Input: part model. Units: mm. Frame: model coordinates. A direction names the side the tool comes from. Coordinates: 2 decimals unless noted, no trailing zeros. Write each loop counter-clockwise with the first axis right and the second up, starting at its lowest first coordinate (ties: lowest second). Pieces come first, ordered by that corner, then holes. Notation, with made-up numbers: M -17.5,4 L 16.5,4 A33 ccw 16.5,36 Z; hole C 9,-5 d3. An arc over 180 degrees is marked long. Use CSV: the item, a comma, the result in double quotes.
```python
from build123d import *

# Parameters (mm, degrees)
F0_W      = 152.0995497704
F0_H      = 153.0030965805
F1_DEPTH  = 25.4
F2_W      = 137.3413652182
F2_H      = 135.8354389668
F3_DEPTH  = 25.4
F4_W      = 120.4748898745
F4_H      = 118.9689487219
F5_DEPTH  = 25.4
F6_W      = 102.4036556482
F6_H      = 100.8977144957
F7_DEPTH  = 25.4
F8_W      = 81.9229260087
F8_H      = 84.0312317014
F9_DEPTH  = 25.4
F10_W     = 66.863566637
F10_H     = 68.3694928885
F11_DEPTH = 25.4
F12_W     = 51.2018278241
F12_H     = 53.9125055075
F13_DEPTH = 25.4
F14_W     = 34.3353450298
F14_H     = 36.4436469972
F15_DEPTH = 25.4
F15_TAPER = 5
F16_W     = 19.8783595115
F16_H     = 20.1795380563
F17_DEPTH = 25.4
F17_TAPER = 5
F18_W     = 7.8308703378
F18_H     = 6.9273011759
F19_DEPTH = 25.4
F19_TAPER = 5


with BuildPart() as f1:
    # F0 (on Front) → F1 (new body)
    with BuildSketch(Plane.XZ):
        with Locations((-0.150591135, -0.150591135)):
            Rectangle(F0_W, F0_H)
    extrude(amount=F1_DEPTH)

    # F2 (on face) → F3 (join)
    with BuildSketch(Plane.XZ.offset(25.4)):
        Rectangle(F2_W, F2_H)
    extrude(amount=F3_DEPTH)

    # F4 (on face) → F5 (join)
    with BuildSketch(Plane.XZ.offset(50.8)):
        Rectangle(F4_W, F4_H)
    extrude(amount=F5_DEPTH)

    # F6 (on face) → F7 (join)
    with BuildSketch(Plane.XZ.offset(76.2)):
        Rectangle(F6_W, F6_H)
    extrude(amount=F7_DEPTH)

    # F8 (on face) → F9 (join)
    with BuildSketch(Plane.XZ.offset(101.6)):
        Rectangle(F8_W, F8_H)
    extrude(amount=F9_DEPTH)

    # F10 (on face) → F11 (join)
    with BuildSketch(Plane.XZ.offset(127)):
        Rectangle(F10_W, F10_H)
    extrude(amount=F11_DEPTH)

    # F12 (on face) → F13 (join)
    with BuildSketch(Plane.XZ.offset(152.4)):
        Rectangle(F12_W, F12_H)
    extrude(amount=F13_DEPTH)

    # F14 (on face) → F15 (join)
    with BuildSketch(Plane.XZ.offset(177.8)):
        Rectangle(F14_W, F14_H)
    extrude(amount=F15_DEPTH, taper=F15_TAPER)

    # F16 (on face) → F17 (join)
    with BuildSketch(Plane.XZ.offset(203.2)):
        Rectangle(F16_W, F16_H)
    extrude(amount=F17_DEPTH, taper=F17_TAPER)

    # F18 (on face) → F19 (join)
    with BuildSketch(Plane.XZ.offset(228.6)):
        Rectangle(F18_W, F18_H)
    extrude(amount=F19_DEPTH, taper=F19_TAPER)


solid = f1.part
```
1. Section C-C (y = -123). Return loops of the section in (x, z).
Resolved:
outline,"M -40.96,-42.02 L 40.96,-42.02 L 40.96,42.02 L -40.96,42.02 Z"
2. Section A-A (x = -57). Return loops of the section in (y, z).
Resolved:
outline,"M -76.2,-59.48 L -50.8,-59.48 L -50.8,-67.92 L -25.4,-67.92 L -25.4,-76.65 L 0,-76.65 L 0,76.35 L -25.4,76.35 L -25.4,67.92 L -50.8,67.92 L -50.8,59.48 L -76.2,59.48 Z"
3. Section B-B (z = -23.5). Return loops of the section in (x, y), then the cut area to 3 significant figures.
Resolved:
outline,"M -76.2,-25.4 L -68.67,-25.4 L -68.67,-50.8 L -60.24,-50.8 L -60.24,-76.2 L -51.2,-76.2 L -51.2,-101.6 L -40.96,-101.6 L -40.96,-127 L -33.43,-127 L -33.43,-152.4 L -25.6,-152.4 L -25.6,-177.8 L 25.6,-177.8 L 25.6,-152.4 L 33.43,-152.4 L 33.43,-127 L 40.96,-127 L 40.96,-101.6 L 51.2,-101.6 L 51.2,-76.2 L 60.24,-76.2 L 60.24,-50.8 L 68.67,-50.8 L 68.67,-25.4 L 75.9,-25.4 L 75.9,0 L -76.2,0 Z"
area,"18,100 mm^2"
4. Section D-D (x = 22). Return loops of the section in (y, z).
Resolved:
outline,"M -177.8,-26.96 L -152.4,-26.96 L -152.4,-34.18 L -127,-34.18 L -127,-42.02 L -101.6,-42.02 L -101.6,-50.45 L -76.2,-50.45 L -76.2,-59.48 L -50.8,-59.48 L -50.8,-67.92 L -25.4,-67.92 L -25.4,-76.65 L 0,-76.65 L 0,76.35 L -25.4,76.35 L -25.4,67.92 L -50.8,67.92 L -50.8,59.48 L -76.2,59.48 L -76.2,50.45 L -101.6,50.45 L -101.6,42.02 L -127,42.02 L -127,34.18 L -152.4,34.18 L -152.4,26.96 L -177.8,26.96 Z"
5. Material intervals for line 1 (Y direction, x = -1, z = -50.5); line 2 (Z direction, x = 47.5, y = -47.5); line 3 (X direction, y = -111, z = 32.5), sorted ascending. Write a range as [from, to].
Resolved:
line 1,"y = [-76.2, 0]"
line 2,"z = [-67.92, 67.92]"
line 3,"x = [-40.96, 40.96]"
6. Contact query for flat-ended pins moving along their axis: pin 1 Ø12.5 at (x, y) = (-15.5, -86) entering from -Z; pin 2 Ø7.5 at (y, z) = (-134, -6) entering from +X; pin 3 Ø12.5 at (y, z) = (-143.5, 1.5) entering from -X. Output: stop coordinate, or through.
Resolved:
pin 1,"stops at z = -50.45"
pin 2,"stops at x = 33.43"
pin 3,"stops at x = -33.43"
7. Access query for faces 1 (the flat face through (-40.961, -114, -1)), 2 (the flat face through (51.202, -89, -1)), 3 (the flat face through (0, -140, -34.185)). Directions: +Z, -Z, +X, -X, +Y, -Y. A direction counts if a zero-diameter tool reaches every point of the face in a straight line with its end or side. Return the directions, or none.
Resolved:
face 1,"+Z, -Z, -X, -Y"
face 2,"+Z, -Z, +X, -Y"
face 3,"-Z, +X, -X, -Y"
